from build123d import *

# Parameters (mm, degrees)
F1_DEPTH = 609.6
F2_W     = 293.7587650299
F2_H     = 609.6
F3_DEPTH = 2032
F4_W     = 49.1579873383
F4_H     = 56.1940948486
F5_DEPTH = 165.1
F6_R     = 19.05
F7_DEPTH = 484.2420126617
F9_DEPTH = 293.7587650299


with BuildPart() as f1:
    # F0 (on Front) → F1 (new body)
    with BuildSketch(Plane.XZ):
        Polygon((-1219.2, 0), (0, 0), (-1219.2, 152.4), align=None)
    extrude(amount=F1_DEPTH)

    # F2 (on face) → F3 (join)
    with BuildSketch(Plane(origin=(0, 0, 0), x_dir=(1, 0, 0), z_dir=(0, 0, -1))):
        with Locations((-1366.079382515, 304.8)):
            Rectangle(F2_W, F2_H)
    extrude(amount=-F3_DEPTH)

    # F4 (on face) → F5 (join)
    with BuildSketch(Plane.YZ.offset(-1219.2)):
        with Locations((-571.5, 1930.4)):
            Rectangle(F4_W, F4_H)
        with Locations((-38.1, 1930.4)):
            Rectangle(F4_W, F4_H)
    extrude(amount=F5_DEPTH)

    # F6 (on face) → F7 (join, through all)
    with BuildSketch(Plane(origin=(0, -546.9210063308, 0), x_dir=(-1, 0, 0), z_dir=(0, 1, 0))):
        with Locations((1085.85, 1930.4)):
            Circle(F6_R)
    extrude(amount=F7_DEPTH)

    # F8 (on face) → F9 (cut, through all)
    with BuildSketch(Plane.YZ.offset(-1219.2)):
        with BuildLine():
            Line((-508, 558.8), (-508, 152.4))
            Line((-508, 152.4), (-101.6, 152.4))
            Line((-101.6, 152.4), (-101.6, 558.8))
            ThreePointArc((-101.6, 558.8), (-304.8, 762), (-508, 558.8))
        make_face()
    extrude(amount=-F9_DEPTH, mode=Mode.SUBTRACT)


solid = f1.part
The listing builds one solid part. Answer for the finished solid, in the listing's coordinates (mm). A direction names the side the tool comes from. Give positions to 0.01 mm unless a question says otherwise; leave off trailing zeros. Loops run counter-clockwise (first coordinate to the right, second up) from the corner with the lowest first, then second, coordinate; pieces in that order, holes last. Notation, with made-up numbers: (5.25, 6.5) - (63.25, 6.5) arc R21 cw to (63.25, 37.5) - close; hole circle Ø2 at (-17, 67). An arc over 180 degrees is marked (long way). Answer as a JSON object with one key per item and string values.
1. A cutting plane is placed at A-A (y = -304.8). Write down the section's boundary in (x, z), then the cut area to 3 significant figures.
Determined:
{"outline": "(-1512.96, 0) - (0, 0) - (-1219.2, 152.4) - (-1512.96, 152.4) - close; (-1512.96, 762) - (-1219.2, 762) - (-1219.2, 2032) - (-1512.96, 2032) - close; circle Ø38.1 at (-1085.85, 1930.4)", "area": "512,000 mm²"}
2. A cutting plane is placed at C-C (z = 786). Write down the section's boundary in (x, y).
Determined:
{"outline": "(-1512.96, -609.6) - (-1219.2, -609.6) - (-1219.2, 0) - (-1512.96, 0) - close"}
3. Find the intervals of material crossed by L1, parallel to X at y = -382.5, z = 1928.5; L2, parallel to X at y = -112, z = 1850; L3, parallel to Y at x = -1278, z = 704.5, in increasing order. Write a range as [from, to].
Determined:
{"L1": "[-1512.96, -1219.2], [-1104.81, -1066.89]", "L2": "[-1512.96, -1219.2]", "L3": "[-609.6, -446.44], [-163.16, 0]"}
4. For faces 1 (the flat face through (-1364, -101.6, 353)), 2 (the flat face through (-1138, -38, 1958.497)), 3 (the flat face through (-1138, -13.521, 1930)), 4 (the flat face through (-1138, -596.079, 1930)), determine the directions among +Z, -Z, +X, -X, +Y, -Y from which every point of the face is accessible in a straight line to the end or side of a thin tool.
Determined:
{"face 1": "+X, -X", "face 2": "+Z, +X, +Y, -Y", "face 3": "+Z, +X, +Y", "face 4": "+Z, +X, -Y"}
5. A cutting plane is placed at B-B (y = -210). Write down the section's boundary in (x, z), then the cut area to 3 significant figures.
Determined:
{"outline": "(-1512.96, 0) - (0, 0) - (-1219.2, 152.4) - (-1512.96, 152.4) - close; (-1512.96, 738.53) - (-1219.2, 738.53) - (-1219.2, 2032) - (-1512.96, 2032) - close; circle Ø38.1 at (-1085.85, 1930.4)", "area": "519,000 mm²"}
6. For a pull along Z with two mould halves and no side action, classify faces 5 (the flat face through (-767, -309, 0)), 6 (the cylindrical face through (-1364.02, -300.33, 761.95)), 7 (the flat face through (-1320, 0, 936)) as pulls with the +Z half, pulls with the -Z half, needs draft (parallel to the pull), parting line crosses it, or undercut.
Determined:
{"face 5": "pulls with the -Z half", "face 6": "undercut", "face 7": "needs draft"}
7. Flat-ended cylindrical pins translate along their axes: pin 1 Ø12 at (y, z) = (-227, 1769) entering from +X; pin 2 Ø14.5 at (y, z) = (-576.5, 1939.5) entering from +X; pin 3 Ø24.5 at (x, y) = (-1145, -45) entering from -Z; pin 4 Ø24.5 at (x, y) = (-1096.5, -48.5) entering from +Z. Find the tip coordinate at first contact, or state that the pin passes through.
Determined:
{"pin 1": "x = -1219.2", "pin 2": "x = -1054.1", "pin 3": "z = 0", "pin 4": "z = 1958.5"}
